```python
from build123d import *

# Parameters (mm, degrees)
CROQUIS3_R            = 2.25
CORTAR_EXTRUIR1_DEPTH = 28.955321497


with BuildPart() as part:
    # Croquis2 → Revolución2 (revolve)
    with BuildSketch(Plane.XY, mode=Mode.PRIVATE) as revoluci_n2_sk:
        with BuildLine():
            ThreePointArc((4.5, -2.875), (2.46221445, -1.397517486), (0, -0.875))
            Line((0, -0.875), (0, -13))
            ThreePointArc((0, -13), (2.46221445, -12.477482514), (4.5, -11))
            Line((4.5, -11), (4.5, -2.875))
        make_face()
        with BuildLine():
            ThreePointArc((6.0625, -6.9375), (5.658407738, -4.761189332), (4.5, -2.875))
            Line((4.5, -2.875), (4.5, -11))
            ThreePointArc((4.5, -11), (5.658407738, -9.113810668), (6.0625, -6.9375))
        make_face()
        with BuildLine():
            Line((4.5, 0), (0, 0))
            Line((0, 0), (0, -0.875))
            ThreePointArc((0, -0.875), (2.46221445, -1.397517486), (4.5, -2.875))
            Line((4.5, -2.875), (4.5, 0))
        make_face()
        with BuildLine():
            Line((17.5, 0), (4.5, 0))
            Line((4.5, 0), (4.5, -2.875))
            ThreePointArc((4.5, -2.875), (5.658407738, -4.761189332), (6.0625, -6.9375))
            ThreePointArc((6.0625, -6.9375), (5.658407738, -9.113810668), (4.5, -11))
            ThreePointArc((4.5, -11), (8.024807813, -7.532680371), (10, -3))
            Line((10, -3), (17.5, -3))
            Line((17.5, -3), (17.5, 0))
        make_face()
    revolve(revoluci_n2_sk.sketch.rotate(Axis((0, 0, 0), (0, -1, 0)), 90), axis=Axis((0, 0, 0), (0, -1, 0)))

    # Croquis3 → Cortar-Extruir1 (cut, through all)
    with BuildSketch(Plane(origin=(0, 0, 0), x_dir=(1, 0, 0), z_dir=(0, 1, 0))):
        with Locations(Location((14, 0, 0), (0, 0, 270))):
            Circle(CROQUIS3_R)
        with Locations(Location((-14, 0, 0), (0, 0, 270))):
            Circle(CROQUIS3_R)
    extrude(amount=-CORTAR_EXTRUIR1_DEPTH, mode=Mode.SUBTRACT)


solid = part.part
```
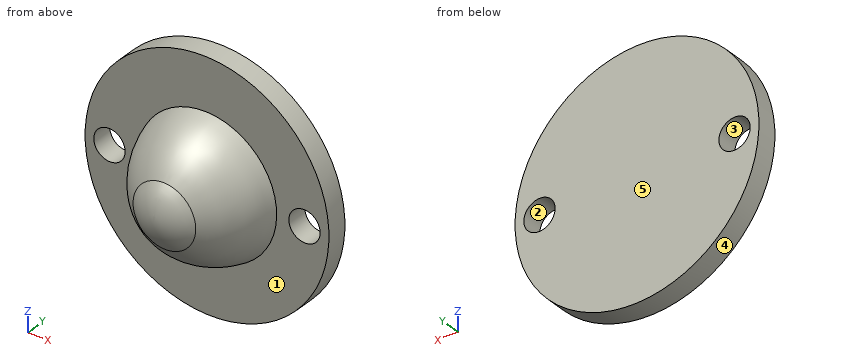
Can you work these out from the model? Positions are in its coordinate system, mm. Face numbers are marked on the shaded views. A direction names the side the tool comes from. Coordinates: 2 decimals unless noted, no trailing zeros. Write each loop counter-clockwise with the first axis right and the second up, starting at its lowest first coordinate (ties: lowest second). Pieces come first, ordered by that corner, then holes. Notation, with made-up numbers: (11.5, 63.5) - (35.5, 63.5) arc R20 ccw to (35.5, 96.5) - close; hole circle Ø9 at (7.5, 73.25). An arc over 180 degrees is marked (long way). Return JSON: item names as keys, results as strings.
Q1. If we section it at A-A (x = 14): Please give me the cut outline in (y, z), then the cut area to 3 significant figures.
Computed values:
{"outline": "(-3, -10.5) - (0, -10.5) - (0, -2.25) - (-3, -2.25) - close; (-3, 2.25) - (0, 2.25) - (0, 10.5) - (-3, 10.5) - close", "area": "49.5 mm2"}
Q2. On a 3-axis mill with a long thin cutter (end or side, diameter ignored), from which of +Z, -Z, +X, -X, +Y, -Y can I reach the whole of each face in a straight line? I mean the marked faces 1 and 2. Say none if no direction works.
Computed values:
{"face 1": "-Y", "face 2": "+Y, -Y"}
Q3. I'm going to push flat-ended pins straight in: pin 1 Ø3 at (x, y) = (7, -5) entering from -Z; pin 2 Ø7 at (x, z) = (14, 0) entering from +Y; pin 3 Ø5 at (x, z) = (-7, 12.5) entering from -Y; pin 4 Ø4 at (x, y) = (6.5, -2.5) entering from +Z. Where does each tip first touch, or does it pass through?
Computed values:
{"pin 1": "stops at z = -7.79", "pin 2": "stops at y = 0", "pin 3": "stops at y = -3", "pin 4": "stops at z = 16.91"}
Q4. If we section it at B-B (y = -2.5): Please give me the cut outline in (x, z), then the cut area to 3 significant figures.
Computed values:
{"outline": "circle Ø35 at (0, 0); hole circle Ø4.5 at (-14, 0); hole circle Ø4.5 at (14, 0)", "area": "930 mm2"}
Q5. Thinking about a two-plate mould opening in X: for the marked faces 3, 4 and 5, which applies, +X half, -X half, draft (parallel to the pull), parting line (faces both ways), or undercut?
Computed values:
{"face 3": "undercut", "face 4": "parting line", "face 5": "draft"}
Q6. If we section it at D-D (z = -14): Please give me the cut outline in (x, y), then the cut area to 3 significant figures.
Computed values:
{"outline": "(-10.5, -3) - (10.5, -3) - (10.5, 0) - (-10.5, 0) - close", "area": "63.0 mm2"}
Q7. Please list where these lines run through material, in increasing order: L1, parallel to X at y = -1.8, z = 0; L2, parallel to Y at x = 3, z = 14; L3, parallel to Z at x = 7.5, y = -4.75. Write a range as from..to.
Computed values:
{"L1": "x = -17.5..-16.25, -11.75..11.75, 16.25..17.5", "L2": "y = -3..0", "L3": "z = -5.79..5.79"}
Q8. If we section it at C-C (z = 0): Count the separate pieces of the cut face and the enclosed holes in it, then the cut area to 3 significant figures.
Computed values:
{"separate pieces": "3", "enclosed holes": "0", "area": "219 mm2"}
